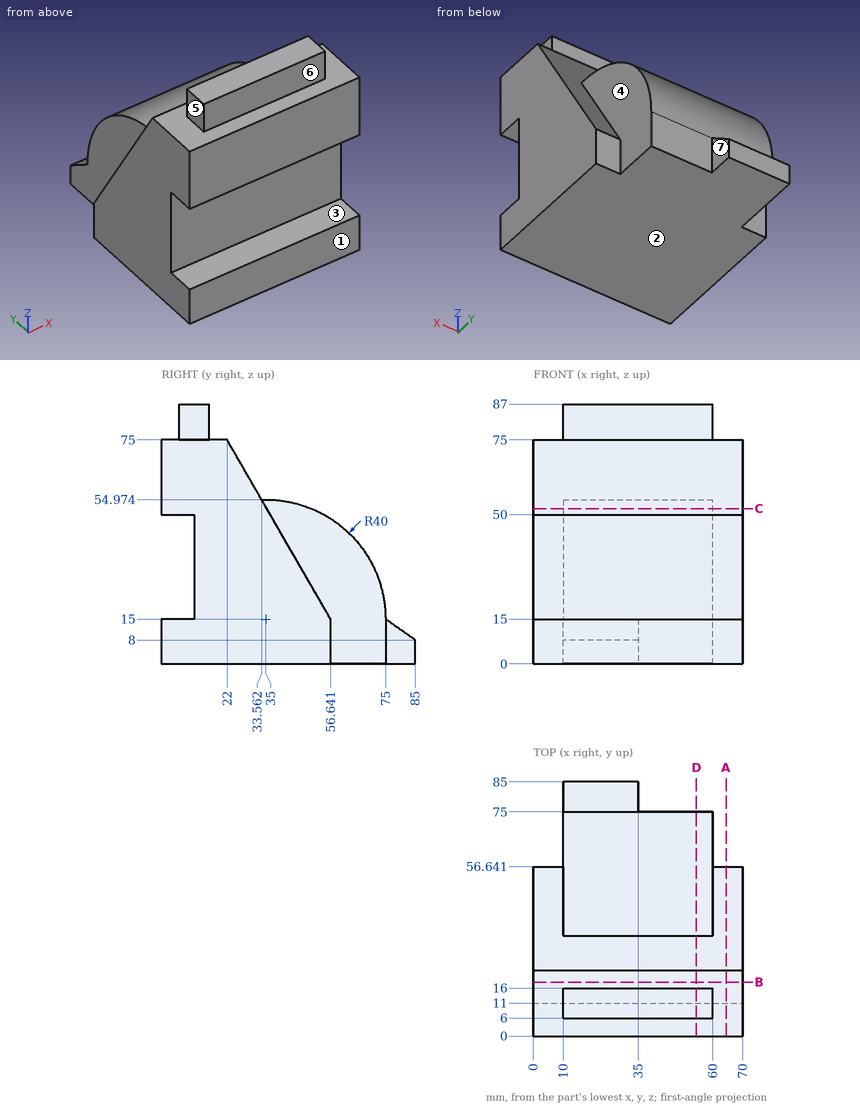
Can you work these out from the drawing? Everything is in mm from the part's minimum corner. A direction names the side the tool comes from. Coordinates: 2 decimals unless noted, no trailing zeros. Loops run counter-clockwise (first coordinate to the right, second up) from the corner with the lowest first, then second, coordinate; pieces in that order, holes last.
1) Will these pins go through, and if not, where does the flat tip stop? pin 1 Ø8 at (x, z) = (40.5, 9.5) entering from +Y; pin 2 Ø17.5 at (x, z) = (36.5, 33) entering from -Y; pin 3 Ø1.5 at (x, z) = (26, 13.5) entering from +Y (1 decimal).
Reported:
pin 1: stops at y = 75
pin 2: stops at y = 11
pin 3: stops at y = 78.2
2) Please list where these lines run through material, in increasing order: line 1 along Z through (x, y) = (26, 6.5); line 2 along X through (y, z) = (53, 41); line 3 along Z through (x, y) = (47.5, 4.5).
Reported:
line 1: z = 0 to 15, 50 to 87
line 2: x = 10 to 60
line 3: z = 0 to 15, 50 to 75
3) Thinking about a two-plate mould opening in Z: for the marked faces 1, 2 and 3, which applies, released by +Z, released by -Z, zero draft, split by the parting line, or undercut?
Reported:
face 1: zero draft
face 2: released by -Z
face 3: undercut
4) Imagine slicing it at C-C (z = 52). List the corners of the cut face in (x, y) for me, and give its area (3 significant figures).
Reported:
outline: (0, 0) - (70, 0) - (70, 35.28) - (60, 35.28) - (60, 50.2) - (10, 50.2) - (10, 35.28) - (0, 35.28) - close
area: 3,220 mm2
5) Imagine slicing it at B-B (y = 18). List the corners of the cut face in (x, z) for me.
Reported:
outline: (0, 0) - (70, 0) - (70, 75) - (0, 75) - close
6) Which directions (+Z, -Z, +X, -X, +Y, -Y) give clear straight access to the entire face, cutting with the end or side of a thin tool? Please do the marked faces 4, 5, 6 and 7.
Reported:
face 4: +Z, +X, +Y
face 5: +Z, -X, +Y, -Y
face 6: +Z, +X, -X, -Y
face 7: +Z, -Z, +X, +Y
7) Imagine slicing it at A-A (x = 64.5). List the corners of the cut face in (y, z) for me.
Reported:
outline: (0, 0) - (56.64, 0) - (56.64, 15) - (22, 75) - (0, 75) - (0, 50) - (11, 50) - (11, 15) - (0, 15) - close
8) Imagine slicing it at D-D (x = 54.5). List the corners of the cut face in (y, z) for me.
Reported:
outline: (0, 0) - (75, 0) - (75, 15) arc R40 ccw to (33.56, 54.97) - (22, 75) - (16, 75) - (16, 87) - (6, 87) - (6, 75) - (0, 75) - (0, 50) - (11, 50) - (11, 15) - (0, 15) - close
